from build123d import *

# Parameters (mm, degrees)
F1_DEPTH = 17.78
F2_SIZE  = 6.35
F4_D     = 3.2766


with BuildPart() as f1:
    # F0 (on Front) → F1 (new body)
    with BuildSketch(Plane.XZ):
        with BuildLine():
            Line((0, 68.2752), (0, 0))
            Line((0, 0), (7.9502, 0))
            Line((7.9502, 0), (7.9502, 47.1932))
            ThreePointArc((7.9502, 47.1932), (13.068568, 59.550032), (25.4254, 64.6684))
            Line((25.4254, 64.6684), (38.1127, 64.6684))
            Line((38.1127, 64.6684), (38.1127, 68.2752))
            Line((38.1127, 68.2752), (0, 68.2752))
        make_face()
    extrude(amount=F1_DEPTH)

    # F2
    f2_edges = [f1.edges().sort_by_distance(p)[0] for p in [
        (0, -8.89, 68.2752),
    ]]
    chamfer(f2_edges, length=F2_SIZE)

    # F4 (through all)
    with Locations(Plane.XZ.offset(17.78)):
        with Locations((12.7, 64.2874), (3.9624, 9.525), (3.9624, 34.925)):
            Hole(F4_D / 2)


solid = f1.part
Geometry check sheet. Reference: the model listing, model coordinates, mm. A direction names the side the tool comes from. Round coordinates to 2 decimals unless told otherwise and drop trailing zeros. Order: outer loops, then holes, each group sorted by start corner. A loop starts at its lowest first (then second) coordinate and runs counter-clockwise, first axis right, second up. Notation, with made-up numbers: (51, -34) -> (70, -34) arc R36 ccw to (70, 0) -> close; hole circle Ø4 at (60, 20). An arc over 180 degrees is marked (long way). Use one line per item in the form item = value.
1. Set-up check for faces 1 (the face through (7.7, 0, 39.4)), 2 (the face through (32, -9, 64.668)): record each of +Z, -Z, +X, -X, +Y, -Y from which the full face is reachable in a straight line by a thin tool's end or side.
Working result:
face_1 = +Z, -Z, +X, -X, +Y
face_2 = -Z, +X, +Y, -Y
2. Go/stop test with flat-tipped pins: pin 1 (1 mm diameter, centred on y = -14.5, z = 35.5, fed in from +X); pin 2 (4 mm diameter, centred on x = 30, y = -16, fed in from -Z); pin 3 (3 mm diameter, centred on x = 12.7, z = 64.29, fed in from -Y). Record where each tip stops, or that it passes through.
Working result:
pin_1 = 7.95
pin_2 = 64.67
pin_3 = through
3. Scan lines: line 1 along Z through (x, y) = (2.5, -1.75); line 2 along X through (y, z) = (-1.25, 13); line 3 along Z through (x, y) = (12.7, -8). Record each from-to range of solid material in increasing order. Write a range as from..to.
Working result:
line_1 = 0..8.79, 10.26..34.19, 35.66..64.43
line_2 = 0..7.95
line_3 = 59.17..62.65, 65.93..68.28
4. Cross-section at A-A, the plane x = 12.7. Enter the section's corners in (y, z), plus the area to 3 significant figures.
Working result:
outline = (-17.78, 59.17) -> (0, 59.17) -> (0, 62.65) -> (-17.78, 62.65) -> close; (-17.78, 65.93) -> (0, 65.93) -> (0, 68.28) -> (-17.78, 68.28) -> close
area = 104 mm^2
5. Cross-section at C-C, the plane z = 30. Enter the section's corners in (x, y).
Working result:
outline = (0, -17.78) -> (7.95, -17.78) -> (7.95, 0) -> (0, 0) -> close
6. Mould release check, pull along X, two halves, no side actions. Record for faces 3 (the face through (3.219, -8.766, 65.145)), 4 (the face through (7.7, -17.78, 39.4)), 5 (the face through (11.944, -8.766, 62.834)): pulls with the +X half, pulls with the -X half, needs draft (parallel to the pull), parting line crosses it, or undercut.
Working result:
face_3 = pulls with the -X half
face_4 = needs draft
face_5 = undercut
7. Cross-section at B-B, the plane y = -6.5. Enter the section's corners in (x, z) (3 decimals).
Working result:
outline = (0, 0) -> (7.95, 0) -> (7.95, 47.193) arc R17.475 cw to (25.425, 64.668) -> (38.113, 64.668) -> (38.113, 68.275) -> (6.35, 68.275) -> (0, 61.925) -> close; hole circle Ø3.277 at (3.962, 9.525); hole circle Ø3.277 at (3.962, 34.925); hole circle Ø3.277 at (12.7, 64.287)
8. Cross-section at D-D, the plane x = 28. Enter the section's corners in (y, z).
Working result:
outline = (-17.78, 64.67) -> (0, 64.67) -> (0, 68.28) -> (-17.78, 68.28) -> close
